```python
from build123d import *

# Parameters (mm, degrees)
CHAMFER_SIZE = 0.12


with BuildPart() as part:
    # Sketch → Revolution (revolve)
    with BuildSketch(Plane.XZ):
        Polygon((-2.78, 3), (-0.8, 3), (-0.8, -1.53), (-2.045, -1.53), (-2.045, 0), (-2.78, 0), align=None)
    revolve(axis=Axis((0, 0, 0), (0, 0, 1)))

    # Chamfer
    chamfer_edges = [part.edges().sort_by_distance(p)[0] for p in [
        (2.78, 0, 3),
        (0.8, 0, 3),
        (2.78, 0, 0),
        (2.045, 0, -1.53),
        (0.8, 0, -1.53),
    ]]
    chamfer(chamfer_edges, length=CHAMFER_SIZE)


solid = part.part
```
Model file for the job. Use its own axes, mm. A direction names the side the tool comes from. Coordinates: 2 decimals unless noted, no trailing zeros. Order: outer loops, then holes, each group sorted by start corner. A loop starts at its lowest first (then second) coordinate and runs counter-clockwise, first axis right, second up. Notation, with made-up numbers: (-39.75, 5) -> (-20.75, 5) arc R19 ccw to (-20.75, 41) -> close; hole circle Ø8 at (9, 89.5). An arc over 180 degrees is marked (long way). Answer as a JSON object with one key per item and string values. Group by question number.
1) Which spindle directions (+Z, -Z, +X, -X, +Y, -Y) get a long thin tool onto all of the face, cutting with end or side? Do faces 1 (the face through (-1, 2, 0)), 2 (the face through (2.2, 1.7, 1.5)). Say none if no direction does.
2) Cut at C-C, the plane z = 2.45. Write the cut outline in (x, y).
3) Pull direction Y, two halves, no side cores. Call faces 3 (the face through (-1.95, -0.61, -0.7)), 4 (the face through (0.63, 0.49, 0.7)), 5 (the face through (-1.1, 0, 3)): +Y half, -Y half, draft (parallel to the pull), parting line (faces both ways), or undercut.
4) Drill centre lines: L1, parallel to Y at x = 0, z = -0.5 (3 decimals); L2, parallel to X at y = 0, z = 1.7. Where is each one in solid material? Low to high.
5) Flat gauge pins, fed straight in: pin 1 (1.4 mm diameter, centred on x = 0, y = 0, fed in from -Z); pin 2 (1 mm diameter, centred on x = -1.5, z = 1, fed in from -Y). Where does each tip first touch, or does it go through?
6) Cut at A-A, the plane x = 0. Write the cut outline in (y, z) (3 decimals), then the cut area to 3 significant figures.
Check values:
{
 "1": {"face 1": "-Z", "face 2": "+Z, -Z"},
 "2": {"outline": "circle Ø5.56 at (0, 0); hole circle Ø1.6 at (0, 0)"},
 "3": {"face 3": "parting line", "face 4": "undercut", "face 5": "draft"},
 "4": {"L1": "y = -2.045 to -0.8, 0.8 to 2.045", "L2": "x = -2.78 to -0.8, 0.8 to 2.78"},
 "5": {"pin 1": "passes through", "pin 2": "stops at y = -2.59"},
 "6": {"outline": "(-2.78, 0.12) -> (-2.66, 0) -> (-2.045, 0) -> (-2.045, -1.41) -> (-1.925, -1.53) -> (-0.92, -1.53) -> (-0.8, -1.41) -> (-0.8, 2.88) -> (-0.92, 3) -> (-2.66, 3) -> (-2.78, 2.88) -> close; (0.8, -1.41) -> (0.92, -1.53) -> (1.925, -1.53) -> (2.045, -1.41) -> (2.045, 0) -> (2.66, 0) -> (2.78, 0.12) -> (2.78, 2.88) -> (2.66, 3) -> (0.92, 3) -> (0.8, 2.88) -> close", "area": "15.6 mm²"}
}
